The listing builds one solid part. Answer for the finished solid, in the listing's coordinates (mm). Round coordinates to 2 decimals unless told otherwise and drop trailing zeros. Loops run counter-clockwise (first coordinate to the right, second up) from the corner with the lowest first, then second, coordinate; pieces in that order, holes last. Notation, with made-up numbers: (-10.5, 70.25) - (1.5, 70.25) arc R35 cw to (1.5, 105.25) - close; hole circle Ø9 at (-16.5, 67). An arc over 180 degrees is marked (long way). Write item = value, one per line. Start each with the question number.
1) Section B-B, the plane x = 111 is taken. Determine the outline of the cut face in (y, z).
2) Given pin 1 Ø1.5 at (x, y) = (85.5, -3) entering from -Z; pin 2 Ø3 at (x, y) = (214.5, -3) entering from +Z; pin 3 Ø1.9 at (y, z) = (-2.5, 189.5) entering from -X; pin 4 Ø4 at (x, z) = (53.19, -117.77) entering from -Y, each flat-ended and moving along its own axis, determine where each tip first touches the part or whether it passes through.
3) Section A-A, the plane y = -1.5 is taken. Give the number of separate pieces and of enclosed holes in the cut face, and give its area (3 significant figures).
4) Section C-C, the plane z = 51.5 is taken. Determine the outline of the cut face in (x, y).
5) Straight lines are drawn through the part: line 1 along Z through (x, y) = (315.5, -3.25); line 2 along Z through (x, y) = (164.5, -0.5); line 3 along X through (y, z) = (-4.5, 170.5). For each, find the intervals that lie inside material, in ascending order.
from build123d import *

# Parameters (mm, degrees)
F0_R     = 2.4765
F1_DEPTH = 6.35


with BuildPart() as f1:
    # F0 (on Front) → F1 (new body)
    with BuildSketch(Plane.XZ):
        with BuildLine():
            Line((-182.687491, 165.680151), (-182.687491, -178.108265))
            ThreePointArc((-182.687491, -178.108265), (-180.680274, -182.741055), (-175.927573, -184.44502))
            ThreePointArc((-175.927573, -184.44502), (68.064874, -138.02089), (293.317944, -33.385482))
            ThreePointArc((293.317944, -33.385482), (327.11409, -7.064195), (342.855905, 32.775295))
            ThreePointArc((342.855905, 32.775295), (342.704473, 35.012459), (341.784916, 37.057514))
            Line((341.784916, 37.057514), (308.354903, 85.916741))
            ThreePointArc((308.354903, 85.916741), (306.076721, 87.947579), (303.114203, 88.680997))
            Line((303.114203, 88.680997), (228.528813, 88.680997))
            Line((228.528813, 88.680997), (228.528813, 108.399421))
            Line((228.528813, 108.399421), (192.847848, 108.399421))
            Line((192.847848, 108.399421), (192.847848, 172.030151))
            Line((192.847848, 172.030151), (-60.674842, 172.030151))
            Line((-60.674842, 172.030151), (-176.337491, 172.030151))
            ThreePointArc((-176.337491, 172.030151), (-180.827619, 170.170279), (-182.687491, 165.680151))
        make_face()
        with Locations((-153.386965, -157.20512)):
            Circle(F0_R, mode=Mode.SUBTRACT)
        with Locations((-55.309255, -144.247517)):
            Circle(F0_R, mode=Mode.SUBTRACT)
        with Locations((53.187076, -117.768265)):
            Circle(F0_R, mode=Mode.SUBTRACT)
        with Locations((-156.203881, -35.138641)):
            Circle(F0_R, mode=Mode.SUBTRACT)
        with Locations((0, -33.260699)):
            Circle(F0_R, mode=Mode.SUBTRACT)
        with Locations((190.371348, -71.606256)):
            Circle(F0_R, mode=Mode.SUBTRACT)
        with Locations((-125.036161, 125.164057)):
            Circle(F0_R, mode=Mode.SUBTRACT)
        with Locations((-162.50541, 154.822963)):
            Circle(F0_R, mode=Mode.SUBTRACT)
        with Locations((-82.966307, 154.368845)):
            Circle(F0_R, mode=Mode.SUBTRACT)
        with Locations((316.099495, 13.687949)):
            Circle(F0_R, mode=Mode.SUBTRACT)
        with BuildLine():
            Line((-60.674842, 205.46418), (-60.674842, 172.030151))
            Line((-60.674842, 172.030151), (192.847848, 172.030151))
            Line((192.847848, 172.030151), (192.847848, 205.46418))
            ThreePointArc((192.847848, 205.46418), (190.987976, 209.954308), (186.497848, 211.81418))
            Line((186.497848, 211.81418), (-54.324842, 211.81418))
            ThreePointArc((-54.324842, 211.81418), (-58.814971, 209.954308), (-60.674842, 205.46418))
        make_face()
        with Locations((-42.673801, 201.054353)):
            Circle(F0_R, mode=Mode.SUBTRACT)
        with Locations((18.518413, 185.048574)):
            Circle(F0_R, mode=Mode.SUBTRACT)
        with Locations((95.800146, 202.318219)):
            Circle(F0_R, mode=Mode.SUBTRACT)
        with Locations((165.061638, 184.351559)):
            Circle(F0_R, mode=Mode.SUBTRACT)
    extrude(amount=F1_DEPTH)


solid = f1.part
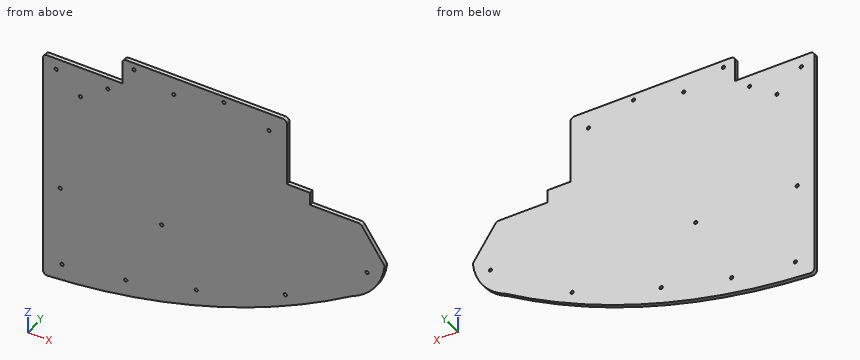
Geometry check:
q1.outline = (-6.35, -123.12) - (0, -123.12) - (0, 211.81) - (-6.35, 211.81) - close
q2.pin_1 = -132.49
q2.pin_2 = 108.4
q2.pin_3 = -60.67
q2.pin_4 = through
q3.separate_pieces = 1
q3.enclosed_holes = 14
q3.area = 151,000 mm2
q4.outline = (-182.69, -6.35) - (331.9, -6.35) - (331.9, 0) - (-182.69, 0) - close
q5.line_1 = -19.58 to 11.29, 16.09 to 75.47
q5.line_2 = -101.44 to 181.94, 186.76 to 211.81
q5.line_3 = -180.47 to 192.85
